Can you work these out from the model? Positions are in its coordinate system, mm. Round coordinates to 2 decimals unless told otherwise and drop trailing zeros. Write each loop counter-clockwise with the first axis right and the second up, starting at its lowest first coordinate (ties: lowest second). Pieces come first, ordered by that corner, then holes. Notation, with made-up numbers: M 88.5,11.5 L 101.5,11.5 A30 ccw 101.5,50.5 Z; hole C 57.5,77 d9. An arc over 180 degrees is marked long. Use one line per item in the form item = value. Start each with the question number.
```python
from build123d import *

# Parameters (mm, degrees)
SKETCH2_R             = 7.6
BOSS_EXTRUDE1_DEPTH   = 19.05
BOSS_EXTRUDE1_2_DEPTH = 19.05
SKETCH3_W             = 141.7
SKETCH3_H             = 33.75
BOSS_EXTRUDE2_DEPTH   = 12.7
BOSS_EXTRUDE3_REACH   = 78.533
CHAMFER2_SIZE         = 1.5875


with BuildPart() as part:
    # Sketch2 → Boss-Extrude1 (new body)
    with BuildSketch(Plane(origin=(0, 0, 0), x_dir=(1, 0, 0), z_dir=(0, 1, 0))):
        with Locations(Location((-50.8, 0, 0), (0, 0, 90))):
            Circle(SKETCH2_R)
    extrude(amount=BOSS_EXTRUDE1_DEPTH)



with BuildPart() as body_2:
    # Sketch2 → Boss-Extrude1 2 (new body)
    with BuildSketch(Plane(origin=(0, 0, 0), x_dir=(1, 0, 0), z_dir=(0, 1, 0))):
        with Locations(Location((50.8, 0, 0), (0, 0, 90))):
            Circle(SKETCH2_R)
    extrude(amount=BOSS_EXTRUDE1_2_DEPTH)


with BuildPart() as part_1:
    add(part.part)

    add(body_2.part)  # Boss-Extrude2 merges body 2
    # Sketch3 → Boss-Extrude2 (add)
    with BuildSketch(Plane(origin=(0, 5.650833475, 8.701520484), x_dir=(-1, 0, 0), z_dir=(0, 0.5446390350150281, 0.8386705679454234))):
        with Locations((0, -15.976674319)):
            Rectangle(SKETCH3_W, SKETCH3_H)
    extrude(amount=BOSS_EXTRUDE2_DEPTH)

    # Sketch8 → Boss-Extrude3 (add, up to next)
    with BuildSketch(Plane(origin=(0, 19.05, 0), x_dir=(1, 0, 0), z_dir=(0, 1, 0)), mode=Mode.PRIVATE) as boss_extrude3_sk1:
        with BuildLine():
            Line((43.2, 0), (58.4, 0))
            ThreePointArc((58.4, 0), (50.8, 7.6), (43.2, 0))
        make_face()
    boss_extrude3_tool1 = extrude(boss_extrude3_sk1.sketch, amount=BOSS_EXTRUDE3_REACH, mode=Mode.PRIVATE) - part_1.part
    # Sketch8 → Boss-Extrude3 (add, up to next)
    with BuildSketch(Plane(origin=(0, 19.05, 0), x_dir=(1, 0, 0), z_dir=(0, 1, 0)), mode=Mode.PRIVATE) as boss_extrude3_sk2:
        with BuildLine():
            ThreePointArc((-43.2, 0), (-50.8, 7.6), (-58.4, 0))
            Line((-58.4, 0), (-43.2, 0))
        make_face()
    boss_extrude3_tool2 = extrude(boss_extrude3_sk2.sketch, amount=BOSS_EXTRUDE3_REACH, mode=Mode.PRIVATE) - part_1.part
    add(boss_extrude3_tool1.solids().sort_by_distance((50.8, 19.05, -3.22554))[0])
    add(boss_extrude3_tool2.solids().sort_by_distance((-50.8, 19.05, -3.22554))[0])

    # Chamfer2
    chamfer2_edges = [part_1.edges().sort_by_distance(p)[0] for p in [
        (70.85, 19.05, 0),
        (0, 4.897434166, 9.190783716),
        (0, 33.202565834, -9.190783716),
        (70.85, 36.661023706, -3.865225609),
        (-70.85, 19.05, 0),
        (-70.85, 36.661023706, -3.865225609),
        (-70.85, 8.355892038, 14.516341822),
        (70.85, 8.355892038, 14.516341822),
    ]]
    chamfer(chamfer2_edges, length=CHAMFER2_SIZE)


solid = part_1.part
```
1. If we section it at B-B (y = 8.5): List the corners of the cut face in (x, z) for me, and give its area (3 significant figures).
2. Will these pins go through, and if not, where does the flat tip stop? pin 1 (3 mm diameter, centred on x = -15.5, y = 8.5, fed in from +Z); pin 2 (6 mm diameter, centred on x = 7, z = 9.5, fed in from +Y); pin 3 (12 mm diameter, centred on y = 31.5, z = 16.5, fed in from +X); pin 4 (3 mm diameter, centred on x = -7.5, y = 35.5, fed in from +Z).
3. If we section it at A-A (x = 29): List the corners of the cut face in (y, z) for me.
4. Please list where these lines run through material, in increasing order: line 1 along X through (y, z) = (3.5, 7); line 2 along X through (y, z) = (16.5, -5.75); line 3 along Z through (x, y) = (57, 9).
5. If we mould it in two halves opening along X, with no side actions, what happens to faces 1 (the face through (0.97, 18.871, 0.117)), 2 (the face through (70.07, 19.67, 0.56)), 3 (the face through (-70.07, 19.67, 0.56))? For each: pulls with the +X half, pulls with the -X half, needs draft (parallel to the pull), parting line crosses it, or undercut.
6. If we section it at D-D (y = 28): List the corners of the cut face in (x, z) for me, and give its area (3 significant figures).
7. If we section it at C-C (x = -53): List the corners of the cut face in (y, z) for me.
Model answer:
q1.outline = M -70.85,8.74 L -69.26,6.85 L -54.09,6.85 A7.6 ccw long -47.51,6.85 L 47.51,6.85 A7.6 ccw long 54.09,6.85 L 69.26,6.85 L 70.85,8.74 L 70.85,11.82 L 69.26,14.74 L -69.26,14.74 L -70.85,11.82 Z
q1.area = 1,470 mm2
q2.pin_1 = 17.05
q2.pin_2 = 32.36
q2.pin_3 = through
q2.pin_4 = 5.43
q3.outline = M 5.76,10.52 L 6.23,8.33 L 31.87,-8.33 L 34.07,-7.86 L 40.12,1.46 L 11.81,19.84 Z
q4.line_1 = -53.76 to -47.84, 47.84 to 53.76
q4.line_2 = -55.77 to -45.83, 45.83 to 55.77
q4.line_3 = -4.4 to 4.4, 6.53 to 15.51
q5.face_1 = undercut
q5.face_2 = pulls with the +X half
q5.face_3 = pulls with the -X half
q6.outline = M -70.85,-3.92 L -69.26,-5.81 L -55.7,-5.81 A7.6 ccw -45.9,-5.81 L 45.9,-5.81 A7.6 ccw 55.7,-5.81 L 69.26,-5.81 L 70.85,-3.92 L 70.85,9.33 L -70.85,9.33 Z
q6.area = 2,170 mm2
q7.outline = M 0,-7.27 L 30.25,-7.27 L 31.87,-8.33 L 34.07,-7.86 L 40.12,1.46 L 11.81,19.84 L 5.76,10.52 L 6.23,8.33 L 7.85,7.27 L 0,7.27 Z
